Part model, mm, in its own coordinate system. A direction names the side the tool comes from. Give positions to 0.01 mm unless a question says otherwise; leave off trailing zeros. Write each loop counter-clockwise with the first axis right and the second up, starting at its lowest first coordinate (ties: lowest second). Pieces come first, ordered by that corner, then holes.
```python
from build123d import *

# Parameters (mm, degrees)
SKETCH_W   = 53
SKETCH_H   = 53
SKETCH_R   = 1.65
SKETCH_R_2 = 3.15
PAD_DEPTH  = 4


with BuildPart() as part:
    # Sketch → Pad (new body)
    with BuildSketch(Plane.XY):
        with Locations((26.5, -26.5)):
            Rectangle(SKETCH_W, SKETCH_H)
        with Locations((2.5, -2.5)):
            Circle(SKETCH_R, mode=Mode.SUBTRACT)
        with Locations((50.5, -2.5)):
            Circle(SKETCH_R, mode=Mode.SUBTRACT)
        with Locations((50.5, -50.5)):
            Circle(SKETCH_R, mode=Mode.SUBTRACT)
        with Locations((2.5, -50.5)):
            Circle(SKETCH_R, mode=Mode.SUBTRACT)
        with Locations((11.5, -11.5)):
            Circle(SKETCH_R_2, mode=Mode.SUBTRACT)
        with Locations((41.5, -11.5)):
            Circle(SKETCH_R_2, mode=Mode.SUBTRACT)
        with Locations((41.5, -41.5)):
            Circle(SKETCH_R_2, mode=Mode.SUBTRACT)
        with Locations((11.5, -41.5)):
            Circle(SKETCH_R_2, mode=Mode.SUBTRACT)
        with BuildLine():
            ThreePointArc((6.601021, -12.5), (15.035534, -15.035534), (12.5, -6.601021))
            Line((40.5, -6.601021), (12.5, -6.601021))
            ThreePointArc((40.5, -6.601021), (37.964466, -15.035534), (46.398979, -12.5))
            Line((46.398979, -40.5), (46.398979, -12.5))
            ThreePointArc((46.398979, -40.5), (37.964466, -37.964466), (40.5, -46.398979))
            Line((12.5, -46.398979), (40.5, -46.398979))
            ThreePointArc((12.5, -46.398979), (15.035534, -37.964466), (6.601021, -40.5))
            Line((6.601021, -12.5), (6.601021, -40.5))
        make_face(mode=Mode.SUBTRACT)
    extrude(amount=PAD_DEPTH)


solid = part.part
```
1) Two-plate mould, pull along X, no slides. Class faces 1 (the face through (10.817, -44.575, 1.972)), 2 (the face through (26, 0, 2)), 3 (the face through (53, -27, 2)): +X half, -X half, draft (parallel to the pull), parting line (faces both ways), or undercut.
Answers follow:
face 1: undercut
face 2: draft
face 3: +X half
2) Saw through at C-C, the plane z = 1.55. Count the separate pieces of the cut face and the enclosed holes in it, then the cut area to 3 significant figures.
Answers follow:
separate pieces: 1
enclosed holes: 9
area: 1,400 mm2
3) Saw through at A-A, the plane x = 11.5. Write the cut outline in (y, z).
Answers follow:
outline: (-53, 0) - (-44.65, 0) - (-44.65, 4) - (-53, 4) - close; (-38.35, 0) - (-36.5, 0) - (-36.5, 4) - (-38.35, 4) - close; (-16.5, 0) - (-14.65, 0) - (-14.65, 4) - (-16.5, 4) - close; (-8.35, 0) - (0, 0) - (0, 4) - (-8.35, 4) - close
4) Pin check, flat tips, straight feed: pin 1 Ø4 at (x, y) = (2.5, -2.5) entering from +Z; pin 2 Ø2 at (x, y) = (50.5, -50.5) entering from -Z. Stop position of each tip, or through.
Answers follow:
pin 1: stops at z = 4
pin 2: passes through
5) Saw through at D-D, the plane y = -50.5. Write the cut outline in (x, z).
Answers follow:
outline: (0, 0) - (0.85, 0) - (0.85, 4) - (0, 4) - close; (4.15, 0) - (48.85, 0) - (48.85, 4) - (4.15, 4) - close; (52.15, 0) - (53, 0) - (53, 4) - (52.15, 4) - close
6) Saw through at B-B, the plane y = -34.5. Write the cut outline in (x, z), then the cut area to 3 significant figures.
Answers follow:
outline: (0, 0) - (6.6, 0) - (6.6, 4) - (0, 4) - close; (46.4, 0) - (53, 0) - (53, 4) - (46.4, 4) - close
area: 52.8 mm2
7) 3-axis set-ups, long thin cutter, end or side, ignore diameter. For faces 4 (the face through (26, -46.399, 2)), 5 (the face through (14, -14, 4)): which of +Z, -Z, +X, -X, +Y, -Y reach the whole face in a straight line?
Answers follow:
face 4: +Z, -Z
face 5: +Z, +X, -X, +Y, -Y
8) Wall check: L1, parallel to Y at x = 11.5, z = 1.25; L2, parallel to Y at x = 2.5, z = 2.95; L3, parallel to Y at x = 49, z = 0.3. Give the ranges that are in metal, low to high.
Answers follow:
L1: y = -53 to -44.65, -38.35 to -36.5, -16.5 to -14.65, -8.35 to 0
L2: y = -53 to -52.15, -48.85 to -4.15, -0.85 to 0
L3: y = -53 to -51.19, -49.81 to -3.19, -1.81 to 0
